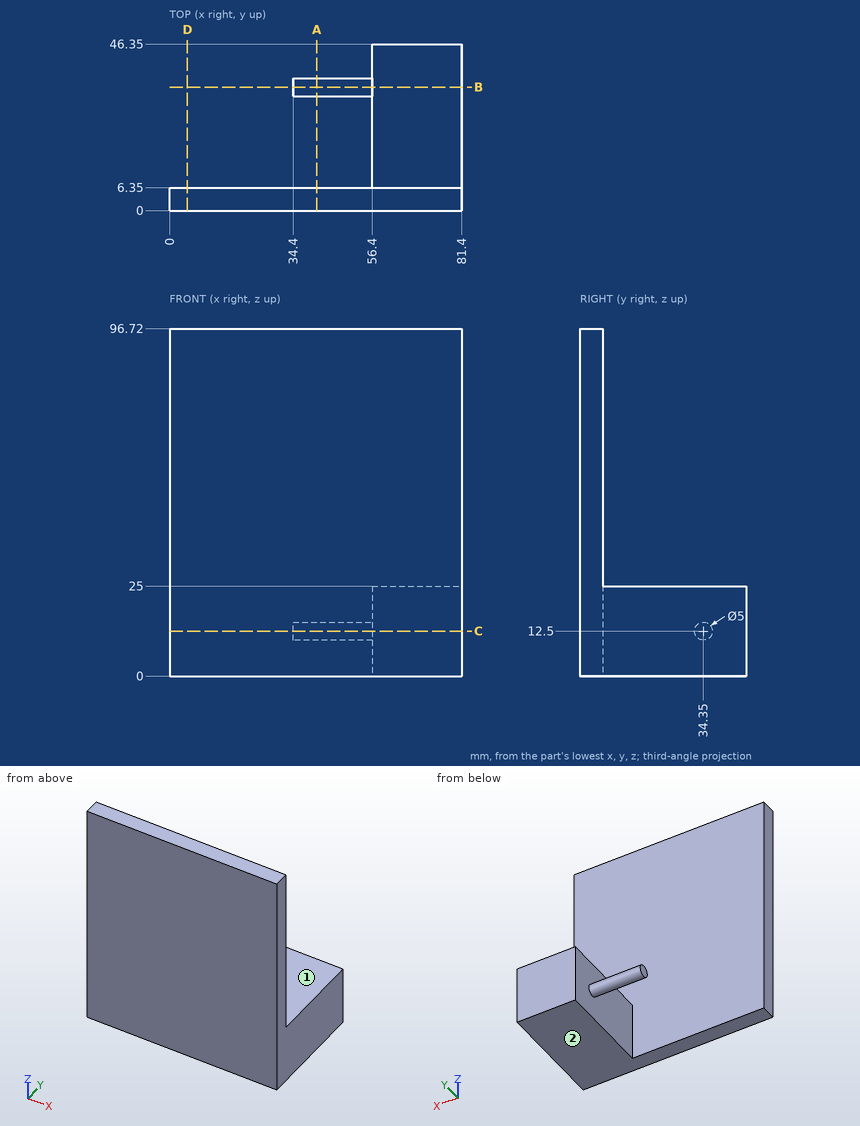
The figure shows three views and two pictorial views of one solid part (mm, origin at its lowest corner). Answer the questions. A direction names the side the tool comes from. Coordinates: 2 decimals unless noted, no trailing zeros. Order: outer loops, then holes, each group sorted by start corner. A loop starts at its lowest first (then second) coordinate and runs counter-clockwise, first axis right, second up.
Q1. A cutting plane is placed at A-A, the plane x = 41. Write down the section's boundary in (y, z), and give its area (3 significant figures).
Q2. Which of the six approach directions +Z, -Z, +X, -X, +Y, -Y give full straight-line access (tool end or side, diameter ignored) to the marked faces 1 and 2?
Q3. A cutting plane is placed at B-B, the plane y = 34.35. Write down the section's boundary in (x, z), and give its area (3 significant figures).
Q4. Consider line 1 (Z direction, x = 72.5, y = 42); line 2 (Y direction, x = 28, z = 77.5); line 3 (X direction, y = 36, z = 16.5). Determine where each line is inside the solid, lowest interval first.
Q5. Given P1, Ø12.5, axis at y = 26, z = 16, coming from the -X side; P2, Ø3, axis at x = 63, y = 28, coming from the +Z side; P3, Ø2, axis at x = 51, y = 32, coming from the -Z side, each flat-ended and moving along its own axis, determine where each tip first touches the part or whether it passes through.
Q6. A cutting plane is placed at C-C, the plane z = 12.5. Write down the section's boundary in (x, y), and give its area (3 significant figures).
Q7. A cutting plane is placed at D-D, the plane x = 5. Write down the section's boundary in (y, z).
Answers follow:
1. outline: (0, 0) - (6.35, 0) - (6.35, 96.72) - (0, 96.72) - close; circle Ø5 at (34.35, 12.5)
1. area: 634 mm2
2. face 1: +Z, +X, -X, +Y
2. face 2: -Z, +X, -X, +Y, -Y
3. outline: (34.4, 10) - (56.4, 10) - (56.4, 0) - (81.4, 0) - (81.4, 25) - (56.4, 25) - (56.4, 15) - (34.4, 15) - close
3. area: 735 mm2
4. line 1: z = 0 to 25
4. line 2: y = 0 to 6.35
4. line 3: x = 56.4 to 81.4
5. P1: stops at x = 56.4
5. P2: stops at z = 25
5. P3: stops at z = 10.4
6. outline: (0, 0) - (81.4, 0) - (81.4, 46.35) - (56.4, 46.35) - (56.4, 36.85) - (34.4, 36.85) - (34.4, 31.85) - (56.4, 31.85) - (56.4, 6.35) - (0, 6.35) - close
6. area: 1,630 mm2
7. outline: (0, 0) - (6.35, 0) - (6.35, 96.72) - (0, 96.72) - close
